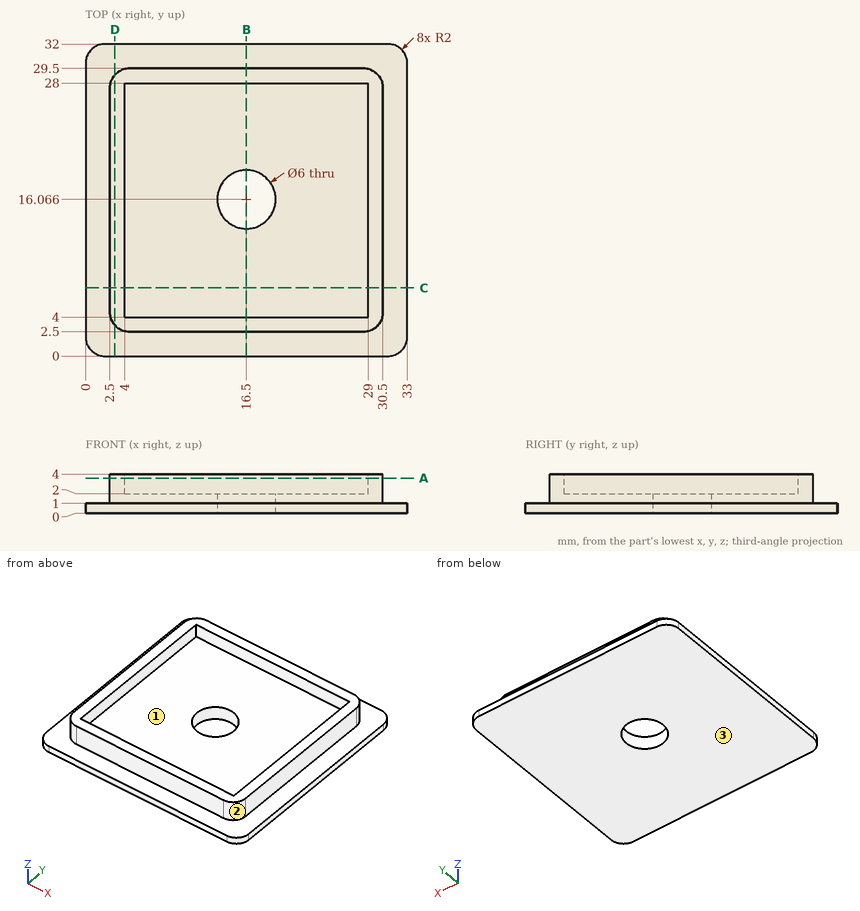
Design review of the part shown in the three views and the two pictorial views. Dimensions are in mm from the part's minimum x, y and z. Round coordinates to 2 decimals unless told otherwise and drop trailing zeros. Order: outer loops, then holes, each group sorted by start corner. A loop starts at its lowest first (then second) coordinate and runs counter-clockwise, first axis right, second up. Notation, with made-up numbers: (-3, 43) - (6, 43) arc R26 cw to (6, 61) - close; hole circle Ø3 at (43.5, 58.5). An arc over 180 degrees is marked (long way). One line per question, with ' | ' between items.
Item 1: For P1, Ø1.6, axis at y = 15.5, z = 3, coming from the +X side; P2, Ø1, axis at x = 10, y = 23, coming from the +Z side; P3, Ø1.5, axis at y = 12, z = 2.5, coming from the -X side, all flat-tipped, find the tip position at first contact; note any pin that passes through.
Checks:
P1: x = 30.5 | P2: z = 2 | P3: x = 2.5
Item 2: Wall thickness on line 1 (X direction, y = 9, z = 2.15); line 2 (Y direction, x = 16.5, z = 1.45); line 3 (Y direction, x = 9, z = 3.4): over which ranges is each line inside the solid? List them lowest first. Write a range as [from, to].
Checks:
line 1: [2.5, 4], [29, 30.5] | line 2: [2.5, 13.07], [19.07, 29.5] | line 3: [2.5, 4], [28, 29.5]
Item 3: Draft analysis for pull direction Y (two halves, no side actions). For the marked faces 1, 2 and 3, state which applies: +Y half, -Y half, draft (parallel to the pull), parting line (faces both ways), or undercut.
Checks:
face 1: undercut | face 2: -Y half | face 3: draft
Item 4: Take a section at B-B, the plane x = 16.5. Write out the cut boundary in (y, z), then the cut area to 3 significant figures.
Checks:
outline: (0, 0) - (13.07, 0) - (13.07, 2) - (4, 2) - (4, 4) - (2.5, 4) - (2.5, 1) - (0, 1) - close; (19.07, 0) - (32, 0) - (32, 1) - (29.5, 1) - (29.5, 4) - (28, 4) - (28, 2) - (19.07, 2) - close | area: 53.0 mm²
Item 5: Take a section at D-D, the plane x = 3. Write out the cut boundary in (y, z).
Checks:
outline: (0, 0) - (32, 0) - (32, 1) - (28.82, 1) - (28.82, 4) - (3.18, 4) - (3.18, 1) - (0, 1) - close
Item 6: Take a section at C-C, the plane y = 7. Write out the cut boundary in (x, z), then the cut area to 3 significant figures.
Checks:
outline: (0, 0) - (33, 0) - (33, 1) - (30.5, 1) - (30.5, 4) - (29, 4) - (29, 2) - (4, 2) - (4, 4) - (2.5, 4) - (2.5, 1) - (0, 1) - close | area: 67.0 mm²
Item 7: Take a section at A-A, the plane z = 3.6. Write out the cut boundary in (x, y), then the cut area to 3 significant figures.
Checks:
outline: (2.5, 4.5) arc R2 ccw to (4.5, 2.5) - (28.5, 2.5) arc R2 ccw to (30.5, 4.5) - (30.5, 27.5) arc R2 ccw to (28.5, 29.5) - (4.5, 29.5) arc R2 ccw to (2.5, 27.5) - close; hole (4, 4) - (29, 4) - (29, 28) - (4, 28) - close | area: 153 mm²
